from build123d import *

# Parameters (mm, degrees)
ESBO_O1_W                = 23
ESBO_O1_H                = 43
RESSALTO_EXTRUS_O1_DEPTH = 8.5
ESBO_O2_W                = 21
ESBO_O2_H                = 33
CORTE_EXTRUS_O1_DEPTH    = 6.1
ESBO_O3_R                = 9.25
CORTE_EXTRUS_O2_DEPTH    = 26.821502667
ESBO_O4_R                = 1
CORTE_EXTRUS_O3_DEPTH    = 4


with BuildPart() as part:
    # Esboço1 → Ressalto-extrusão1 (new body)
    with BuildSketch(Plane.XY):
        Rectangle(ESBO_O1_W, ESBO_O1_H)
    extrude(amount=RESSALTO_EXTRUS_O1_DEPTH)

    # Esboço2 → Corte-extrusão1 (cut)
    with BuildSketch(Plane(origin=(0, 0, 0), x_dir=(-1, 0, 0), z_dir=(0, 0, -1))):
        Rectangle(ESBO_O2_W, ESBO_O2_H)
    extrude(amount=-CORTE_EXTRUS_O1_DEPTH, mode=Mode.SUBTRACT)

    # Esboço3 → Corte-extrusão2 (cut, through all)
    with BuildSketch(Plane.XY.offset(8.5)):
        Circle(ESBO_O3_R)
    extrude(amount=-CORTE_EXTRUS_O2_DEPTH, mode=Mode.SUBTRACT)

    # Esboço4 → Corte-extrusão3 (cut)
    with BuildSketch(Plane(origin=(0, 0, 0), x_dir=(-1, 0, 0), z_dir=(0, 0, -1))):
        with Locations((0, 19)):
            Circle(ESBO_O4_R)
        with Locations(Location((0, -19, 0), (0, 0, 180))):
            Circle(ESBO_O4_R)
    extrude(amount=-CORTE_EXTRUS_O3_DEPTH, mode=Mode.SUBTRACT)


solid = part.part
Source: CAD feature listing. Evaluate the final solid. Frame: model axes, mm. A direction names the side the tool comes from. Give positions to 0.01 mm unless a question says otherwise; leave off trailing zeros. Write each loop counter-clockwise with the first axis right and the second up, starting at its lowest first coordinate (ties: lowest second). Pieces come first, ordered by that corner, then holes. Notation, with made-up numbers: (81, 45) - (137, 45) arc R12 ccw to (137, 61) - close; hole circle Ø3 at (76.25, -35.75). An arc over 180 degrees is marked (long way). Write item = value, one per line. Start each with the question number.
Q1. Reachability of faces 5 (the flat face through (-8, 5, 8.5)), 6 (the flat face through (0, -16.5, 3)) from +Z, -Z, +X, -X, +Y, -Y: full face, straight path, thin tool, end or side. Return the list, or none.
Q2. Material intervals for probe 1 along Y at (x, z) = (-3.75, 0.75); probe 2 along Y at (x, z) = (0, 7.6); probe 3 along X at (y, z) = (0, 3.25), sorted ascending.
Q3. Cut plane B-B, the plane z = 4.75. Return loops of the section in (x, y).
Q4. Draft query along X for faces 1 (the cylindrical face through (0, 18, 2)), 2 (the flat face through (10.5, 0, 3)), 3 (the flat face through (11.5, 0, 4)), 4 (the flat face through (0, -21.5, 4)). Return one class per face: +X half, -X half, draft (parallel to the pull), parting line (faces both ways), or undercut.
Q5. Pin query (flat end, axial travel): pin 1 Ø4 at (x, y) = (7.5, -9.5) entering from -Z; pin 2 Ø1 at (x, y) = (0, 19) entering from -Z; pin 3 Ø11 at (x, y) = (0, 0) entering from +Z. Return the tip coordinate at first contact, or that it passes through.
Q6. Cut plane A-A, the plane y = 0. Return loops of the section in (x, z), then the cut area to 3 significant figures.
Q7. Cut plane D-D, the plane y = -16. Return loops of the section in (x, z).
Q8. Cut plane C-C, the plane x = 0. Return loops of the section in (y, z), then the cut area to 3 significant figures.
Computed values:
q1.face_5 = +Z, +X, -X, +Y, -Y
q1.face_6 = -Z
q2.probe_1 = -21.5 to -16.5, 16.5 to 21.5
q2.probe_2 = -21.5 to -9.25, 9.25 to 21.5
q2.probe_3 = -11.5 to -10.5, 10.5 to 11.5
q3.outline = (-11.5, -21.5) - (11.5, -21.5) - (11.5, 21.5) - (-11.5, 21.5) - close; hole (-10.5, -16.5) - (10.5, -16.5) - (10.5, 16.5) - (-10.5, 16.5) - close
q4.face_1 = undercut
q4.face_2 = undercut
q4.face_3 = +X half
q4.face_4 = draft
q5.pin_1 = 6.1
q5.pin_2 = 4
q5.pin_3 = through
q6.outline = (-11.5, 0) - (-10.5, 0) - (-10.5, 6.1) - (-9.25, 6.1) - (-9.25, 8.5) - (-11.5, 8.5) - close; (9.25, 6.1) - (10.5, 6.1) - (10.5, 0) - (11.5, 0) - (11.5, 8.5) - (9.25, 8.5) - close
q6.area = 23.0 mm²
q7.outline = (-11.5, 0) - (-10.5, 0) - (-10.5, 6.1) - (10.5, 6.1) - (10.5, 0) - (11.5, 0) - (11.5, 8.5) - (-11.5, 8.5) - close
q8.outline = (-21.5, 0) - (-20, 0) - (-20, 4) - (-18, 4) - (-18, 0) - (-16.5, 0) - (-16.5, 6.1) - (-9.25, 6.1) - (-9.25, 8.5) - (-21.5, 8.5) - close; (9.25, 6.1) - (16.5, 6.1) - (16.5, 0) - (18, 0) - (18, 4) - (20, 4) - (20, 0) - (21.5, 0) - (21.5, 8.5) - (9.25, 8.5) - close
q8.area = 104 mm²
